Check sheet for the modelled part. Datum: model origin and axes. Units: mm. Face numbers are marked on the shaded views. A direction names the side the tool comes from. Coordinates: 2 decimals unless noted, no trailing zeros. Order: outer loops, then holes, each group sorted by start corner. A loop starts at its lowest first (then second) coordinate and runs counter-clockwise, first axis right, second up.
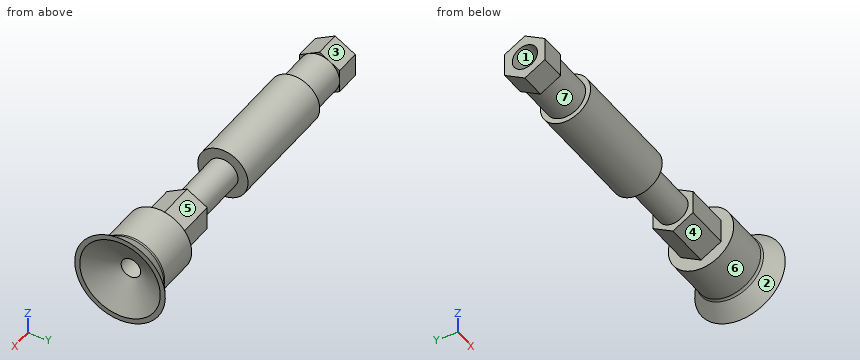
from build123d import *

# Parameters (mm, degrees)
EXTRUDE_1_DEPTH     = 5
SKETCH_2_R          = 4
EXTRUDE_2_DEPTH     = 8
SKETCH_3_R          = 5
EXTRUDE_3_DEPTH     = 23
SKETCH_4_R          = 3
EXTRUDE_4_DEPTH     = 11.5
EXTRUDE_5_DEPTH     = 9
SKETCH_6_R          = 2.5
CUT_EXTRUDE_1_DEPTH = 5
SKETCH_7_R          = 2
CUT_EXTRUDE_2_DEPTH = 8
SKETCH_8_R          = 2.5
CUT_EXTRUDE_3_DEPTH = 45.070965499
SKETCH_9_R          = 6.5
EXTRUDE_6_DEPTH     = 9
FILLET_1_R          = 1
SKETCH_11_R         = 8
CUT_EXTRUDE_4_DEPTH = 3.5
CUT_EXTRUDE_4_DRAFT = -60
CUT_EXTRUDE_START   = -10
SKETCH_12_R         = 2.5
CUT_EXTRUDE_5_DEPTH = 10


with BuildPart() as part:
    # 草图1 → 凸台-拉伸1 (new body)
    with BuildSketch(Plane(origin=(0, 0, 0), x_dir=(0, 0, -1), z_dir=(1, 0, 0))):
        Polygon((2.309401077, 4), (-2.309401077, 4), (-4.618802154, 0), (-2.309401077, -4), (2.309401077, -4), (4.618802154, 0), align=None)
    extrude(amount=EXTRUDE_1_DEPTH)

    # 草图2 → 凸台-拉伸2 (add)
    with BuildSketch(Plane(origin=(5, 0, 0), x_dir=(0, 0, -1), z_dir=(1, 0, 0))):
        with Locations(Location((0, 0, 0), (0, 0, 150))):
            Circle(SKETCH_2_R)
    extrude(amount=EXTRUDE_2_DEPTH)

    # 草图3 → 凸台-拉伸3 (add)
    with BuildSketch(Plane(origin=(13, 0, 0), x_dir=(0, 0, -1), z_dir=(1, 0, 0))):
        Circle(SKETCH_3_R)
    extrude(amount=EXTRUDE_3_DEPTH)

    # 草图4 → 凸台-拉伸4 (add)
    with BuildSketch(Plane(origin=(36, 0, 0), x_dir=(0, 0, -1), z_dir=(1, 0, 0))):
        Circle(SKETCH_4_R)
    extrude(amount=EXTRUDE_4_DEPTH)

    # 草图5 → 凸台-拉伸5 (add)
    with BuildSketch(Plane(origin=(47.5, 0, 0), x_dir=(0, 0, -1), z_dir=(1, 0, 0))):
        Polygon((2.309401077, 4), (-2.309401077, 4), (-4.618802154, 0), (-2.309401077, -4), (2.309401077, -4), (4.618802154, 0), align=None)
    extrude(amount=EXTRUDE_5_DEPTH)

    # 草图6 → 切除-拉伸1 (cut)
    with BuildSketch(Plane.ZY):
        Circle(SKETCH_6_R)
    extrude(amount=-CUT_EXTRUDE_1_DEPTH, mode=Mode.SUBTRACT)

    # 草图7 → 切除-拉伸2 (cut)
    with BuildSketch(Plane.ZY.offset(-5)):
        Circle(SKETCH_7_R)
    extrude(amount=-CUT_EXTRUDE_2_DEPTH, mode=Mode.SUBTRACT)

    # 草图8 → 切除-拉伸3 (cut, through all)
    with BuildSketch(Plane.ZY.offset(-13)):
        Circle(SKETCH_8_R)
    extrude(amount=-CUT_EXTRUDE_3_DEPTH, mode=Mode.SUBTRACT)

    # 草图9 → 凸台-拉伸6 (add)
    with BuildSketch(Plane(origin=(56.5, 0, 0), x_dir=(0, 0, -1), z_dir=(1, 0, 0))):
        Circle(SKETCH_9_R)
    extrude(amount=EXTRUDE_6_DEPTH)

    # 草图10 → 旋转1 (revolve)
    with BuildSketch(Plane(origin=(0, 0, 0), x_dir=(-1, 0, 0), z_dir=(0, 0, -1)), mode=Mode.PRIVATE) as revolve_1_sk:
        Polygon((-65.5, 0), (-69, 0), (-69, 9), (-65.5, 6.5), align=None)
    revolve(revolve_1_sk.sketch.rotate(Axis((65.5, 0, 0), (-1, 0, 0)), 90), axis=Axis((65.5, 0, 0), (-1, 0, 0)))

    # 圆角1
    fillet_1_edges = [part.edges().sort_by_distance(p)[0] for p in [
        (65.5, 0, 6.5),
    ]]
    fillet(fillet_1_edges, radius=FILLET_1_R)


with BuildPart() as cut_extrude_4_tool:
    # 草图11 → 切除-拉伸4 (with draft: the straight prism first)
    with BuildSketch(Plane(origin=(69, 0, 0), x_dir=(0, 0, -1), z_dir=(1, 0, 0))):
        Circle(SKETCH_11_R)
    extrude(amount=-CUT_EXTRUDE_4_DEPTH)
    # 切除-拉伸4: the draft: its side faces are tilted about the plane it starts from
    cut_extrude_4_sides = [cut_extrude_4_tool.faces().sort_by_distance(p)[0] for p in [
        (67.25, 0, 8),
    ]]
    draft(cut_extrude_4_sides, Plane(origin=(69, 0, 0), x_dir=(0, 0, -1), z_dir=(1, 0, 0)), CUT_EXTRUDE_4_DRAFT)


with BuildPart() as part_1:
    add(part.part)

    # 切除-拉伸4: cut by cut_extrude_4_tool
    add(cut_extrude_4_tool.part, mode=Mode.SUBTRACT)

    # 草图12 → 切除-拉伸5 (cut)
    with BuildSketch(Plane(origin=(65.5, 0, 0), x_dir=(0, 0, -1), z_dir=(1, 0, 0)).offset(CUT_EXTRUDE_START)):
        with Locations(Location((0, 0, 0), (0, 0, 180))):
            Circle(SKETCH_12_R)
    extrude(amount=CUT_EXTRUDE_5_DEPTH, mode=Mode.SUBTRACT)


solid = part_1.part
(1) Cross-section at B-B (x = 60.5). Enter the section's corners in (y, z).
Filled in:
outline: circle Ø13 at (0, 0); hole circle Ø5 at (0, 0)
(2) Thickness scan on probe 1 along Y at (x, z) = (1.8, 0); probe 2 along Y at (x, z) = (35, 0); probe 3 along Z at (x, y) = (41.5, -0.5). Record the ranges inside material, lowest first.
Filled in:
probe 1: y = -4 to -2.5, 2.5 to 4
probe 2: y = -5 to -2.5, 2.5 to 5
probe 3: z = -2.96 to -2.45, 2.45 to 2.96
(3) Release check for a two-part mould opening along Z. For the marked faces 1, 2, 3 and 4 record: +Z half, -Z half, draft (parallel to the pull), parting line (faces both ways), or undercut.
Filled in:
face 1: undercut
face 2: parting line
face 3: +Z half
face 4: -Z half
(4) Cross-section at A-A (x = 28). Enter the section's corners in (y, z).
Filled in:
outline: circle Ø10 at (0, 0); hole circle Ø5 at (0, 0)
(5) Go/stop test with flat-tipped pins: P1, Ø3, axis at x = 20, z = -2, coming from the -Y side; P2, Ø3, axis at x = 53, z = -3.5, coming from the +Y side; P3, Ø1, axis at y = -3.5, z = 2.5, coming from the +X side; P4, Ø3, axis at y = 0, z = 0, coming from the +X side. Record where each tip stops, or that it passes through.
Filled in:
P1: stops at y = -4.97
P2: stops at y = 4
P3: stops at x = 67.15
P4: passes through
(6) Tool access check on the marked faces 5, 6 and 7. Record the directions out of +Z, -Z, +X, -X, +Y, -Y that give a thin tool (end or side, any length) a straight path to the whole face; none if there is none.
Filled in:
face 5: +Z, +Y
face 6: -X
face 7: none
